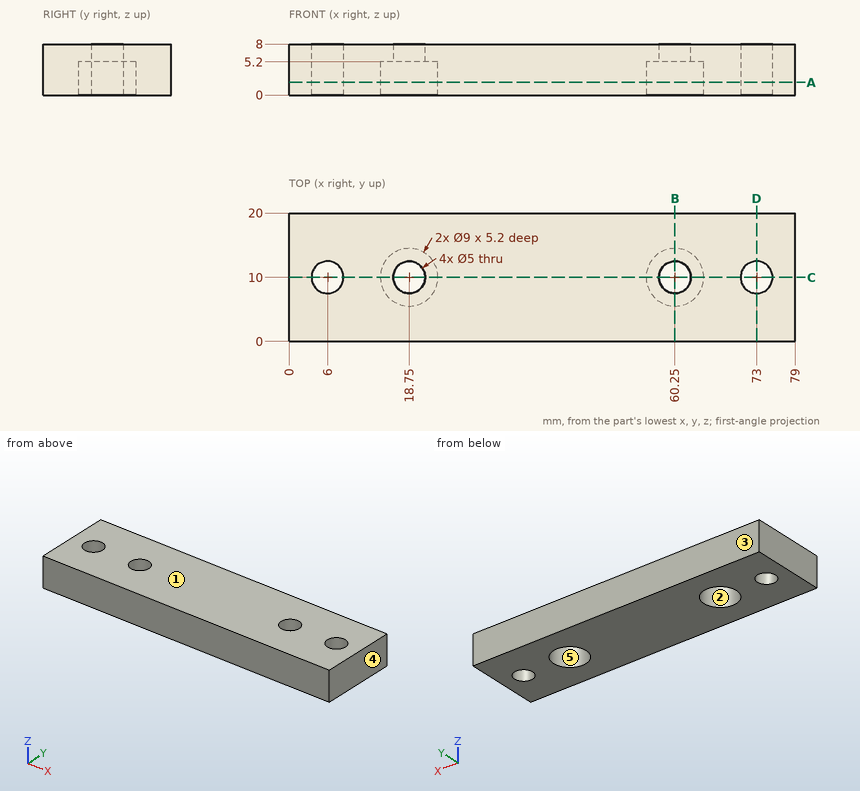
Geometry: see drawing. Coordinates: mm, zero at the bounding-box minimum. A direction names the side the tool comes from. Round coordinates to 2 decimals unless told otherwise and drop trailing zeros. Write each loop counter-clockwise with the first axis right and the second up, starting at its lowest first coordinate (ties: lowest second). Pieces come first, ordered by that corner, then holes.
1) Cut plane D-D (x = 73). Return the cut outline in (y, z).
2) Contact query for a flat-ended pin moving along its axis: P1, Ø8, axis at x = 18.75, y = 10, coming from the -Z side. Output: stop coordinate, or through.
3) Cut plane B-B (x = 60.25). Return the cut outline in (y, z).
4) Cut plane A-A (z = 2). Return the cut outline in (x, y), then the cut area to 3 significant figures.
5) Reachability of the marked faces 1 and 2 from +Z, -Z, +X, -X, +Y, -Y: full face, straight path, thin tool, end or side. Return the list, or none.
6) Cut plane C-C (y = 10). Return the cut outline in (x, z).
7) Draft query along X for the marked faces 3, 4 and 5. Return one class per face: pulls with the +X half, pulls with the -X half, needs draft (parallel to the pull), parting line crosses it, or undercut.
8) Ray query, L1, parallel to Y at x = 64, z = 4.5; L2, parallel to X at y = 11, z = 6; L3, parallel to X at y = 8.5, z = 6.25. Return the intervals inside material, ascending.
Geometry says:
1. outline: (0, 0) - (7.5, 0) - (7.5, 8) - (0, 8) - close; (12.5, 0) - (20, 0) - (20, 8) - (12.5, 8) - close
2. P1: stops at z = 5.2
3. outline: (0, 0) - (5.5, 0) - (5.5, 5.2) - (7.5, 5.2) - (7.5, 8) - (0, 8) - close; (12.5, 5.2) - (14.5, 5.2) - (14.5, 0) - (20, 0) - (20, 8) - (12.5, 8) - close
4. outline: (0, 0) - (79, 0) - (79, 20) - (0, 20) - close; hole circle Ø5 at (6, 10); hole circle Ø9 at (18.75, 10); hole circle Ø9 at (60.25, 10); hole circle Ø5 at (73, 10)
4. area: 1,410 mm2
5. face 1: +Z, +X, -X, +Y, -Y
5. face 2: -Z
6. outline: (0, 0) - (3.5, 0) - (3.5, 8) - (0, 8) - close; (8.5, 0) - (14.25, 0) - (14.25, 5.2) - (16.25, 5.2) - (16.25, 8) - (8.5, 8) - close; (21.25, 5.2) - (23.25, 5.2) - (23.25, 0) - (55.75, 0) - (55.75, 5.2) - (57.75, 5.2) - (57.75, 8) - (21.25, 8) - close; (62.75, 5.2) - (64.75, 5.2) - (64.75, 0) - (70.5, 0) - (70.5, 8) - (62.75, 8) - close; (75.5, 0) - (79, 0) - (79, 8) - (75.5, 8) - close
7. face 3: needs draft
7. face 4: pulls with the +X half
7. face 5: undercut
8. L1: y = 0 to 7.51, 12.49 to 20
8. L2: x = 0 to 3.71, 8.29 to 16.46, 21.04 to 57.96, 62.54 to 70.71, 75.29 to 79
8. L3: x = 0 to 4, 8 to 16.75, 20.75 to 58.25, 62.25 to 71, 75 to 79
